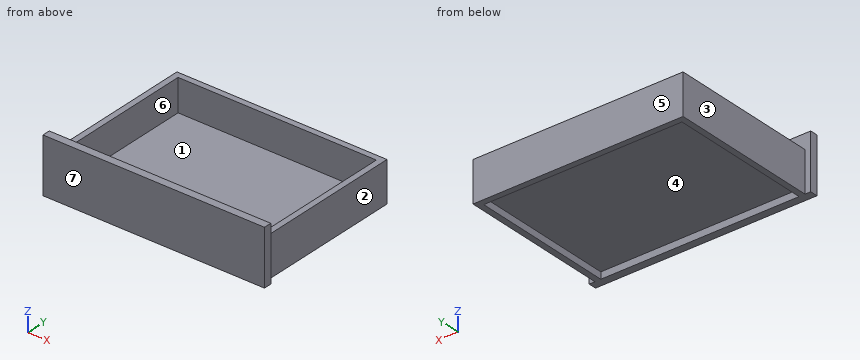
Autodesk Fusion 360 part; units mm, degrees
sketch "Sketch1" plane through (0, 0, 0) normal (0, 0, 1) x (1, 0, 0)
  line L0 (0, 0) -> (407.924, 0)
  line L1 (407.924, 0) -> (407.924, -297.942)
  line L2 (407.924, -297.942) -> (0, -297.942)
  line L3 (0, -297.942) -> (0, 0)
  dimension "d1" = 407.924
  dimension "d2" = 297.942
extrude "Extrude1" add sketch "Sketch1" along normal blind 3.175
sketch "Sketch2" plane through (0, 0, 3.175) normal (0, 0, 1) x (-1, 0, 0)
  line L0 (0, 297.942) -> (-407.924, 297.942)
  line L1 (-407.924, 297.942) -> (-407.924, 0)
  line L2 (-407.924, 0) -> (0, 0)
  line L3 (0, 0) -> (0, 297.942)
  line L4 (-420.074, 297.942) -> (-420.074, -12.15)
  line L5 (-420.074, -12.15) -> (12.15, -12.15)
  line L6 (12.15, -12.15) -> (12.15, 297.942)
  line L7 (0, 297.942) -> (12.15, 297.942)
  line L8 (12.15, 297.942) -> (-420.074, 297.942)
extrude "Extrude2" add sketch "Sketch2" against normal blind 17 contours L1 L2 L3 L4 L5 L6 L7 L8
sketch "Sketch3" plane through (0, 0, 3.175) normal (0, 0, 1) x (-1, 0, 0)
  line L0 (12.15, 297.942) -> (-420.074, 297.942)
  line L1 (-420.074, 297.942) -> (-420.074, -12.15)
  line L2 (-420.074, -12.15) -> (12.15, -12.15)
  line L3 (12.15, -12.15) -> (12.15, 297.942)
  line L4 (-407.924, 285.792) -> (-407.924, 0)
  line L5 (-407.924, 0) -> (0, 0)
  line L6 (0, 0) -> (0, 285.792)
  line L7 (0, 285.792) -> (-407.924, 285.792)
  line L8 (0, 285.792) -> (0, 297.942)
  line L9 (-407.924, 285.792) -> (-407.924, 297.942)
  line L10 (-407.924, 297.942) -> (0, 297.942)
  line L11 (0, 297.942) -> (12.15, 297.942)
  line L12 (12.15, 297.942) -> (12.15, -12.15)
  line L13 (12.15, -12.15) -> (0, -12.15)
  line L14 (-420.074, -12.15) -> (-420.074, 297.942)
  line L15 (-420.074, 297.942) -> (-407.924, 297.942)
  line L16 (-420.074, -12.15) -> (12.15, -12.15)
  dimension "d8" = -12.15
extrude "Extrude3" add sketch "Sketch3" along normal blind 66.15 contours L0 L1 L2 L3 L4 L5 L6 L8 L9 L11 L12 L13 L14 L15 L16
sketch "Sketch4" plane through (0, 0, -13.825) normal (0, 0, -1) x (1, 0, 0)
  line L0 (420.074, 297.942) -> (407.924, 297.942)
  line L1 (407.924, 297.942) -> (407.924, 0)
  line L2 (407.924, 0) -> (0, 0)
  line L3 (0, 0) -> (0, 297.942)
  line L4 (0, 297.942) -> (-12.15, 297.942)
  line L5 (-12.15, 297.942) -> (-12.15, -12.15)
  line L6 (-12.15, -12.15) -> (420.074, -12.15)
  line L7 (420.074, -12.15) -> (420.074, 297.942)
  line L8 (-12.15, 297.942) -> (-23.9, 297.942)
  line L9 (420.074, 297.942) -> (431.824, 297.942)
  line L10 (-23.9, 297.942) -> (-23.9, 313.942)
  line L11 (431.824, 297.942) -> (431.824, 313.942)
  line L12 (-23.9, 313.942) -> (431.824, 313.942)
  line L13 (-12.15, 297.942) -> (420.074, 297.942)
  dimension "d11" = 11.75
  dimension "d12" = 11.75
  dimension "d14" = 16
  dimension "d15" = 16
extrude "Extrude4" add sketch "Sketch4" against normal blind 113.5 contours L0 L4 L8 L9 L10 L11 L12 L13
Input: part model. Units: mm. Frame: model coordinates. Face numbers are marked on the shaded views. A direction names the side the tool comes from. Coordinates: 2 decimals unless noted, no trailing zeros. Loops run counter-clockwise (first coordinate to the right, second up) from the corner with the lowest first, then second, coordinate; pieces in that order, holes last.
(1) Section A-A on z = -6. Return the cut outline in (x, y), then the cut area to 3 significant figures.
(2) Set-up query: the marked faces 1, 2 and 3. Return all of +Z, -Z, +X, -X, +Y, -Y with unobstructed straight access to the full face (end or side cutting, diameter ignored); none if empty.
(3) Section D-D on z = 80. Return the cut outline in (x, y), then the cut area to 3 significant figures.
(4) First-contact query: pin 1 Ø4 at (y, z) = (-139, -6) entering from -X; pin 2 Ø1.5 at (x, y) = (327, -126.5) entering from -Z; pin 3 Ø10 at (x, y) = (113, -126) entering from +Z (3 decimals). Flat tips, straight axial feed; report the tip coordinate or a pass-through.
(5) Section C-C on y = -130.5. Return the cut outline in (x, z) (3 decimals), then the cut area to 3 significant figures.
(6) Material intervals for probe 1 along X at (y, z) = (-211.5, 36.5); probe 2 along Y at (x, z) = (183.5, 46.5); probe 3 along Z at (x, y) = (208.5, -142.5) (3 decimals), sorted ascending.
(7) Pull-direction query (Y, two-part tool) for the marked faces 4, 5, 6 and 7; classes: released by +Y, released by -Y, zero draft, split by the parting line, or undercut.
(8) Section B-B on x = 61.5. Return the cut outline in (y, z) (3 decimals), then the cut area to 3 significant figures.
Data:
1. outline: (-23.9, -313.94) - (431.82, -313.94) - (431.82, -297.94) - (420.07, -297.94) - (420.07, 12.15) - (-12.15, 12.15) - (-12.15, -297.94) - (-23.9, -297.94) - close; hole (0, -297.94) - (407.92, -297.94) - (407.92, 0) - (0, 0) - close
1. area: 19,800 mm2
2. face 1: +Z
2. face 2: +Z, -Z, +X, +Y
2. face 3: +Z, -Z, -X, +Y
3. outline: (-23.9, -313.94) - (431.82, -313.94) - (431.82, -297.94) - (-23.9, -297.94) - close
3. area: 7,290 mm2
4. pin 1: stops at x = -12.15
4. pin 2: stops at z = 0
4. pin 3: stops at z = 3.175
5. outline: (-12.15, -13.825) - (0, -13.825) - (0, 0) - (407.924, 0) - (407.924, -13.825) - (420.074, -13.825) - (420.074, 69.325) - (407.924, 69.325) - (407.924, 3.175) - (0, 3.175) - (0, 69.325) - (-12.15, 69.325) - close
5. area: 3,320 mm2
6. probe 1: x = -12.15 to 0, 407.92 to 420.07
6. probe 2: y = -313.94 to -297.94, 0 to 12.15
6. probe 3: z = 0 to 3.175
7. face 4: undercut
7. face 5: released by +Y
7. face 6: undercut
7. face 7: released by -Y
8. outline: (-313.942, -13.825) - (-297.942, -13.825) - (-297.942, 0) - (0, 0) - (0, -13.825) - (12.15, -13.825) - (12.15, 69.325) - (0, 69.325) - (0, 3.175) - (-297.942, 3.175) - (-297.942, 99.675) - (-313.942, 99.675) - close
8. area: 3,770 mm2
